Check sheet for the modelled part. Datum: model origin and axes. Units: mm. Face numbers are marked on the shaded views. A direction names the side the tool comes from. Coordinates: 2 decimals unless noted, no trailing zeros. Loops run counter-clockwise (first coordinate to the right, second up) from the corner with the lowest first, then second, coordinate; pieces in that order, holes last. Notation, with made-up numbers: M 12.5,35 L 54.5,35 A22 ccw 54.5,49 Z; hole C 69.25,34 d3. An arc over 180 degrees is marked long. Write each question's results on one line, items separated by ' | '. Start each with the question number.
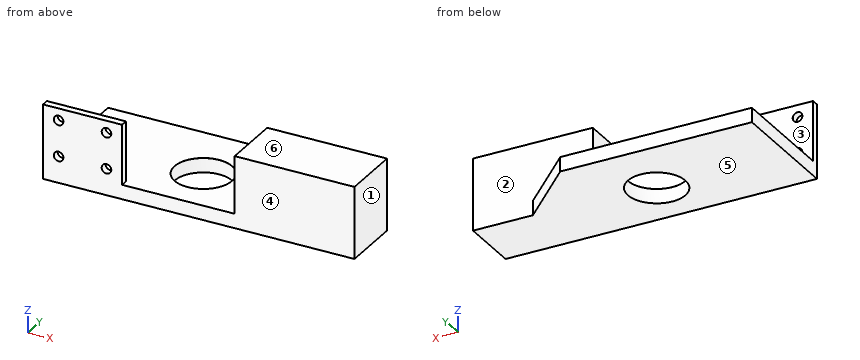
from build123d import *

# Parameters (mm, degrees)
SKETCH1_W                            = 80
SKETCH1_H                            = 80
BOSS_EXTRUDE1_DEPTH                  = 3
SKETCH2_W                            = 33
SKETCH2_H                            = 3
BOSS_EXTRUDE2_DEPTH                  = 25
F_4_0_4_DIAMETER_HOLE1_D             = 4
F_4_0_4_DIAMETER_HOLE1_DEPTH         = 8
F_4_0_4_DIAMETER_HOLE1_CSINK_D       = 4.05
F_4_0_4_DIAMETER_HOLE1_CSINK_ANGLE   = 90
F_4_0_4_DIAMETER_HOLE1_TIP           = 1.201721238
F_24_0_24_DIAMETER_HOLE1_D           = 24
F_24_0_24_DIAMETER_HOLE1_DEPTH       = 8
F_24_0_24_DIAMETER_HOLE1_CSINK_D     = 24.05
F_24_0_24_DIAMETER_HOLE1_CSINK_ANGLE = 90
F_24_0_24_DIAMETER_HOLE1_TIP         = 7.210327428
SKETCH9_W                            = 80
SKETCH9_H                            = 30
CUT_EXTRUDE1_DEPTH                   = 15
SKETCH10_W                           = 50
SKETCH10_H                           = 25
BOSS_EXTRUDE4_DEPTH                  = 30
CHAMFER2_SIZE                        = 25


with BuildPart() as part:
    # Sketch1 → Boss-Extrude1 (new, symmetric)
    with BuildSketch(Plane.XY):
        Rectangle(SKETCH1_W, SKETCH1_H)
    extrude(amount=BOSS_EXTRUDE1_DEPTH, both=True)

    # Sketch2 → Boss-Extrude2 (add)
    with BuildSketch(Plane.XY.offset(3)):
        with Locations((-23.5, -38.5)):
            Rectangle(SKETCH2_W, SKETCH2_H)
    extrude(amount=BOSS_EXTRUDE2_DEPTH)

    # Ø4.0 (4) Diameter Hole1
    with Locations(Plane(origin=(0, -37, 0), x_dir=(1, 0, 0), z_dir=(0, 1, 0))):
        with Locations((-33.5, -8), (-13.5, -8), (-13.5, -23), (-33.5, -23)):
            CounterSinkHole(F_4_0_4_DIAMETER_HOLE1_D / 2, F_4_0_4_DIAMETER_HOLE1_CSINK_D / 2, depth=F_4_0_4_DIAMETER_HOLE1_DEPTH, counter_sink_angle=F_4_0_4_DIAMETER_HOLE1_CSINK_ANGLE)
            with Locations((0, 0, -(F_4_0_4_DIAMETER_HOLE1_DEPTH + F_4_0_4_DIAMETER_HOLE1_TIP / 2))):  # 118° drill point
                Cone(0, F_4_0_4_DIAMETER_HOLE1_D / 2, F_4_0_4_DIAMETER_HOLE1_TIP, mode=Mode.SUBTRACT)

    # Ø24.0 (24) Diameter Hole1
    with Locations(Plane.XY.offset(3)):
        with Locations((15, -18.07)):
            CounterSinkHole(F_24_0_24_DIAMETER_HOLE1_D / 2, F_24_0_24_DIAMETER_HOLE1_CSINK_D / 2, depth=F_24_0_24_DIAMETER_HOLE1_DEPTH, counter_sink_angle=F_24_0_24_DIAMETER_HOLE1_CSINK_ANGLE)
            with Locations((0, 0, -(F_24_0_24_DIAMETER_HOLE1_DEPTH + F_24_0_24_DIAMETER_HOLE1_TIP / 2))):  # 118° drill point
                Cone(0, F_24_0_24_DIAMETER_HOLE1_D / 2, F_24_0_24_DIAMETER_HOLE1_TIP, mode=Mode.SUBTRACT)

    # Sketch9 → Cut-Extrude1 (cut)
    with BuildSketch(Plane.XY.offset(3)):
        with Locations((0, 25)):
            Rectangle(SKETCH9_W, SKETCH9_H)
    extrude(amount=-CUT_EXTRUDE1_DEPTH, mode=Mode.SUBTRACT)

    # Sketch10 → Boss-Extrude4 (add)
    with BuildSketch(Plane(origin=(0, 0, -3), x_dir=(-1, 0, 0), z_dir=(0, 0, -1))):
        with Locations((-65, -27.5)):
            Rectangle(SKETCH10_W, SKETCH10_H)
    extrude(amount=-BOSS_EXTRUDE4_DEPTH)

    # Chamfer2
    chamfer2_edges = [part.edges().sort_by_distance(p)[0] for p in [
        (40, -15, 0),
    ]]
    chamfer(chamfer2_edges, length=CHAMFER2_SIZE - 0.0001)  # a hair under: the kernel refuses the full size


solid = part.part
1) Set-up check for the marked faces 1, 2 and 3: record each of +Z, -Z, +X, -X, +Y, -Y from which the full face is reachable in a straight line by a thin tool's end or side.
2) Section check D-D (y = -18.07). Enter the section's corners in (x, z) (3 decimals).
3) Section check B-B (z = 8). Enter the section's corners in (x, y) (3 decimals), then the cut area to 4 significant figures.
4) Release check for a two-part mould opening along Z. For the marked faces 4, 5 and 6 record: +Z half, -Z half, draft (parallel to the pull), parting line (faces both ways), or undercut.
5) Section check C-C (x = -13.5). Enter the section's corners in (y, z) (3 decimals), then the cut area to 3 significant figures.
6) Section check A-A (x = 15). Enter the section's corners in (y, z) (3 decimals).
7) Thickness scan on probe 1 along X at (y, z) = (-39, 8); probe 2 along Z at (x, y) = (-33.5, -38.65); probe 3 along X at (y, z) = (-18.07, -0.3). Record the ranges inside material, lowest first.
8) Gauge pin test, flat ends, axial feed: P1, Ø7.5, axis at x = 75, y = -29.5, coming from the +Z side; P2, Ø2, axis at y = -23.5, z = 7.5, coming from the -X side; P3, Ø6, axis at x = 25.5, y = -11, coming from the +Z side; P4, Ø19, axis at x = 15, y = -18.07, coming from the +Z side. Record the tip position at first contact, or that the pin passes through.
Return value:
1) face 1: +Z, -Z, +X, +Y, -Y | face 2: +Z, +X, +Y | face 3: +Z, -X, +Y
2) outline: M -40,-3 L 3,-3 L 3,2.975 L 2.975,3 L -40,3 Z; M 27,-3 L 90,-3 L 90,27 L 40,27 L 40,3 L 27.025,3 L 27,2.975 Z
3) outline: M -40,-40 L -35.5,-40 L -35.5,-37.025 L -35.525,-37 L -40,-37 Z; M -31.5,-40 L -15.5,-40 L -15.5,-37.025 L -15.525,-37 L -31.475,-37 L -31.5,-37.025 Z; M -11.5,-40 L -7,-40 L -7,-37 L -11.475,-37 L -11.5,-37.025 Z; M 40,-40 L 90,-40 L 90,-15 L 40,-15 Z | area: 1,325 mm2
4) face 4: draft | face 5: -Z half | face 6: +Z half
5) outline: M -40,-3 L 10,-3 L 10,3 L -37,3 L -37,5.975 L -37.025,6 L -40,6 Z; M -40,10 L -37.025,10 L -37,10.025 L -37,20.975 L -37.025,21 L -40,21 Z; M -40,25 L -37.025,25 L -37,25.025 L -37,28 L -40,28 Z | area: 351 mm2
6) outline: M -40,-3 L -30.07,-3 L -30.07,2.975 L -30.095,3 L -40,3 Z; M -6.07,-3 L 10,-3 L 10,3 L -6.045,3 L -6.07,2.975 Z
7) probe 1: x = -40 to -35.5, -31.5 to -15.5, -11.5 to -7, 40 to 90 | probe 2: z = -3 to 6, 10 to 21, 25 to 28 | probe 3: x = -40 to 3, 27 to 90
8) P1: stops at z = 27 | P2: stops at x = 40 | P3: stops at z = 3 | P4: passes through
